For this review, take the finished solid that the model builds, in its own axes (mm). Face numbers are marked on the shaded views. A direction names the side the tool comes from. Round coordinates to 2 decimals unless told otherwise and drop trailing zeros. Write each loop counter-clockwise with the first axis right and the second up, starting at its lowest first coordinate (ties: lowest second). Pieces come first, ordered by that corner, then holes.
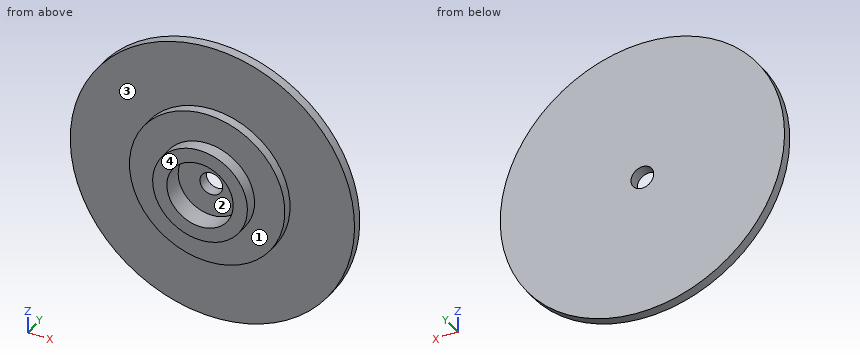
from build123d import *

# Parameters (mm, degrees)
ESQUISSE1_R             = 41
ESQUISSE1_R_2           = 6
BOSS_EXTRU_1_DEPTH      = 10
ESQUISSE2_R             = 17.5
ENL_V_MAT_EXTRU_1_DEPTH = 4
BOSS_EXTRU_2_START      = -5
ESQUISSE3_R             = 75
ESQUISSE3_R_2           = 6
BOSS_EXTRU_2_DEPTH      = 5
BOSS_EXTRU_3_START      = 6.83
ESQUISSE4_R             = 25
ESQUISSE4_R_2           = 17.5
BOSS_EXTRU_3_DEPTH      = 6.83


with BuildPart() as part:
    # Esquisse1 → Boss.-Extru.1 (new body)
    with BuildSketch(Plane(origin=(0, 0, 0), x_dir=(1, 0, 0), z_dir=(0, 1, 0))):
        with Locations(Location((0, 0, 0), (0, 0, 270))):
            Circle(ESQUISSE1_R)
        with Locations(Location((0, 0, 0), (0, 0, 270))):
            Circle(ESQUISSE1_R_2, mode=Mode.SUBTRACT)
    extrude(amount=BOSS_EXTRU_1_DEPTH)

    # Esquisse2 → Enlèv. mat.-Extru.1 (cut)
    with BuildSketch(Plane.XZ):
        with Locations(Location((0, 0, 0), (0, 0, 270))):
            Circle(ESQUISSE2_R)
    extrude(amount=-ENL_V_MAT_EXTRU_1_DEPTH, mode=Mode.SUBTRACT)

    # Esquisse3 → Boss.-Extru.2 (add)
    with BuildSketch(Plane(origin=(0, 10, 0), x_dir=(1, 0, 0), z_dir=(0, 1, 0)).offset(BOSS_EXTRU_2_START)):
        with Locations(Location((0, 0, 0), (0, 0, 270))):
            Circle(ESQUISSE3_R)
        with Locations(Location((0, 0, 0), (0, 0, 90))):
            Circle(ESQUISSE3_R_2, mode=Mode.SUBTRACT)
    extrude(amount=BOSS_EXTRU_2_DEPTH)

    # Esquisse4 → Boss.-Extru.3 (add)
    with BuildSketch(Plane.XZ.offset(BOSS_EXTRU_3_START)):
        with Locations(Location((0, 0, 0), (0, 0, 90))):
            Circle(ESQUISSE4_R)
        with Locations(Location((0, 0, 0), (0, 0, 270))):
            Circle(ESQUISSE4_R_2, mode=Mode.SUBTRACT)
    extrude(amount=-BOSS_EXTRU_3_DEPTH)


solid = part.part
(1) For pin 1 Ø1 at (y, z) = (3.5, 26) entering from +X; pin 2 Ø12 at (x, z) = (-32.5, 39) entering from -Y; pin 3 Ø6 at (x, y) = (6, 4) entering from -Z, all flat-tipped, find the tip position at first contact; note any pin that passes through.
Geometry check:
pin 1: stops at x = 32.11
pin 2: stops at y = 5
pin 3: stops at z = -74.93
(2) For the marked faces 3 and 4, list the 3-axis set-ups (+Z, -Z, +X, -X, +Y, -Y) from which the entire face can be reached by the end or side of a thin tool; tool diameter is ignored.
Geometry check:
face 3: -Y
face 4: +Z, -Z, +X, -X, -Y
(3) We need section A-A, the plane z = 0. Give the boundary of the cut face in (x, y).
Geometry check:
outline: (-75, 5) - (-41, 5) - (-41, 0) - (-25, 0) - (-25, -6.83) - (-17.5, -6.83) - (-17.5, 4) - (-6, 4) - (-6, 10) - (-75, 10) - close; (6, 4) - (17.5, 4) - (17.5, -6.83) - (25, -6.83) - (25, 0) - (41, 0) - (41, 5) - (75, 5) - (75, 10) - (6, 10) - close
(4) We need section B-B, the plane x = 0. Give the boundary of the cut face in (y, z).
Geometry check:
outline: (-6.83, -25) - (0, -25) - (0, -41) - (5, -41) - (5, -75) - (10, -75) - (10, -6) - (4, -6) - (4, -17.5) - (-6.83, -17.5) - close; (-6.83, 17.5) - (4, 17.5) - (4, 6) - (10, 6) - (10, 75) - (5, 75) - (5, 41) - (0, 41) - (0, 25) - (-6.83, 25) - close
(5) Mouldability with a two-part tool opening along X and no side actions: class the marked faces 1 and 2 as pulls with the +X half, pulls with the -X half, needs draft (parallel to the pull), parting line crosses it, or undercut.
Geometry check:
face 1: needs draft
face 2: undercut
(6) For line 1 along X through (y, z) = (6.1, 0); line 2 along X through (y, z) = (-4.5, 0); line 3 along Y through (x, z) = (-37.5, -56.5), list the stretches that pass through material, from the lowest coordinate up.
Geometry check:
line 1: x = -75 to -6, 6 to 75
line 2: x = -25 to -17.5, 17.5 to 25
line 3: y = 5 to 10
(7) We need section D-D, the plane z = 37. Give the boundary of the cut face in (x, y), and give its area (3 significant figures).
Geometry check:
outline: (-65.24, 5) - (-17.66, 5) - (-17.66, 0) - (17.66, 0) - (17.66, 5) - (65.24, 5) - (65.24, 10) - (-65.24, 10) - close
area: 829 mm2
(8) We need section C-C, the plane y = -1.75. Give the boundary of the cut face in (x, z), and give its area (3 significant figures).
Geometry check:
outline: circle Ø50 at (0, 0); hole circle Ø35 at (0, 0)
area: 1,000 mm2
